```python
from build123d import *

# Parameters (mm, degrees)
SALIENTE_EXTRUIR1_DEPTH = 6


with BuildPart() as part:
    # Corte → Saliente-Extruir1 (new body)
    with BuildSketch(Plane.XY):
        Polygon((113.99992211, 146.05), (113.999928646, 140), (86.000028142, 140), (86.000028142, 146.05), (80.000028142, 146.05), (80.000028142, 140), (76.000028142, 140), (76.000028142, 131.000000972), (75.000028142, 130.000001013), (57.20005465, 130.000001734), (56.20005465, 129.000001774), (56.20005465, 71.000001774), (57.20005465, 70.000001734), (75.000028142, 70.000001013), (76.000028142, 69.000000972), (76.000028142, 60), (80.000028142, 60), (80.000028142, 53.95), (86.000028142, 53.95), (86.000028142, 60), (114.00001507, 60), (114.000021606, 53.95), (120.000021606, 53.95), (120.00001507, 60), (124.00001507, 60), (124.000005347, 68.999999028), (125.000004267, 69.999998987), (142.80005465, 69.999998266), (143.80005465, 70.999998226), (143.80005465, 128.999998226), (142.80005465, 129.999998266), (124.999939449, 129.999998987), (123.999938369, 130.999999028), (123.999928646, 140), (119.999928646, 140), (119.99992211, 146.05), align=None)
        Polygon((71.50005465, 126.700001641), (128.50005465, 126.699998845), (128.50005465, 120.699998845), (71.50005465, 120.700001155), align=None, mode=Mode.SUBTRACT)
        Polygon((87.50005465, 73.300000506), (128.50005465, 73.299998359), (128.50005465, 79.299998845), (87.50005465, 79.300000506), align=None, mode=Mode.SUBTRACT)
        with BuildLine():
            add(Edge.make_bspline(
                [(139.147057668, 90.199998471), (139.147059335, 89.428473471), (138.521585686, 88.802997119), (137.750060686, 88.802995452)],
                knots=[0, 0, 0, 0, 1, 1, 1, 1], degree=3))
            add(Edge.make_bspline(
                [(137.750060686, 88.802995452), (136.978535686, 88.802993785), (136.353059335, 89.428467434), (136.353057668, 90.199992434)],
                knots=[0, 0, 0, 0, 1, 1, 1, 1], degree=3))
            add(Edge.make_bspline(
                [(136.353057668, 90.199992434), (136.353056001, 90.971517434), (136.97852965, 91.596993785), (137.75005465, 91.596995452)],
                knots=[0, 0, 0, 0, 1, 1, 1, 1], degree=3))
            add(Edge.make_bspline(
                [(137.75005465, 91.596995452), (138.52157965, 91.596997119), (139.147056001, 90.971523471), (139.147057668, 90.199998471)],
                knots=[0, 0, 0, 0, 1, 1, 1, 1], degree=3))
        make_face(mode=Mode.SUBTRACT)
        with BuildLine():
            add(Edge.make_bspline(
                [(139.147057668, 121.799998471), (139.147059335, 121.028473471), (138.521585686, 120.402997119), (137.750060686, 120.402995452)],
                knots=[0, 0, 0, 0, 1, 1, 1, 1], degree=3))
            add(Edge.make_bspline(
                [(137.750060686, 120.402995452), (136.978535686, 120.402993785), (136.353059335, 121.028467434), (136.353057668, 121.799992434)],
                knots=[0, 0, 0, 0, 1, 1, 1, 1], degree=3))
            add(Edge.make_bspline(
                [(136.353057668, 121.799992434), (136.353056001, 122.571517434), (136.97852965, 123.196993785), (137.75005465, 123.196995452)],
                knots=[0, 0, 0, 0, 1, 1, 1, 1], degree=3))
            add(Edge.make_bspline(
                [(137.75005465, 123.196995452), (138.52157965, 123.196997119), (139.147056001, 122.571523471), (139.147057668, 121.799998471)],
                knots=[0, 0, 0, 0, 1, 1, 1, 1], degree=3))
        make_face(mode=Mode.SUBTRACT)
        with BuildLine():
            add(Edge.make_bspline(
                [(63.647057668, 121.800001529), (63.647059335, 121.028476529), (63.021585686, 120.403000178), (62.250060686, 120.402998511)],
                knots=[0, 0, 0, 0, 1, 1, 1, 1], degree=3))
            add(Edge.make_bspline(
                [(62.250060686, 120.402998511), (61.478535686, 120.402996844), (60.853059335, 121.028470493), (60.853057668, 121.799995493)],
                knots=[0, 0, 0, 0, 1, 1, 1, 1], degree=3))
            add(Edge.make_bspline(
                [(60.853057668, 121.799995493), (60.853056001, 122.571520493), (61.47852965, 123.196996844), (62.25005465, 123.196998511)],
                knots=[0, 0, 0, 0, 1, 1, 1, 1], degree=3))
            add(Edge.make_bspline(
                [(62.25005465, 123.196998511), (63.02157965, 123.197000178), (63.647056001, 122.571526529), (63.647057668, 121.800001529)],
                knots=[0, 0, 0, 0, 1, 1, 1, 1], degree=3))
        make_face(mode=Mode.SUBTRACT)
        with BuildLine():
            add(Edge.make_bspline(
                [(63.647057668, 90.200001529), (63.647059335, 89.428476529), (63.021585686, 88.803000178), (62.250060686, 88.802998511)],
                knots=[0, 0, 0, 0, 1, 1, 1, 1], degree=3))
            add(Edge.make_bspline(
                [(62.250060686, 88.802998511), (61.478535686, 88.802996844), (60.853059335, 89.428470493), (60.853057668, 90.199995493)],
                knots=[0, 0, 0, 0, 1, 1, 1, 1], degree=3))
            add(Edge.make_bspline(
                [(60.853057668, 90.199995493), (60.853056001, 90.971520493), (61.47852965, 91.596996844), (62.25005465, 91.596998511)],
                knots=[0, 0, 0, 0, 1, 1, 1, 1], degree=3))
            add(Edge.make_bspline(
                [(62.25005465, 91.596998511), (63.02157965, 91.597000178), (63.647056001, 90.971526529), (63.647057668, 90.200001529)],
                knots=[0, 0, 0, 0, 1, 1, 1, 1], degree=3))
        make_face(mode=Mode.SUBTRACT)
    extrude(amount=-SALIENTE_EXTRUIR1_DEPTH)


solid = part.part
```
The model under review builds one solid part; all positions refer to its coordinate system, in mm. A direction names the side the tool comes from. Round coordinates to 2 decimals unless told otherwise and drop trailing zeros. Loops run counter-clockwise (first coordinate to the right, second up) from the corner with the lowest first, then second, coordinate; pieces in that order, holes last. Notation, with made-up numbers: M -38,54.5 L 17,54.5 A21 ccw 17,59.5 Z; hole C 66,33 d8. An arc over 180 degrees is marked long. Answer as a JSON object with one key per item and string values.
(1) To check wall thickness, follow line 1 along Y through (x, z) = (62, -5.5); line 2 along Y through (x, z) = (108.5, -1.5); line 3 along Y through (x, z) = (81, -1.75). State the ranges of each line that lie inside material, in increasing order.
Resolved:
{"line 1": "70 to 88.83, 91.57 to 120.43, 123.17 to 130", "line 2": "60 to 73.3, 79.3 to 120.7, 126.7 to 140", "line 3": "53.95 to 120.7, 126.7 to 146.05"}
(2) Clearance check with flat-ended pins moving along their axes: P1, Ø1.8, axis at x = 107.5, z = -3.5, coming from the +Y side; P2, Ø3, axis at y = 56, z = -2.5, coming from the -X side; P3, Ø2, axis at y = 136.5, z = -1.5, coming from the +X side. State where each tip first meets the part, or that it passes through.
Resolved:
{"P1": "y = 140", "P2": "x = 80", "P3": "x = 124"}
(3) Take a section at D-D on y = 138. Give the boundary of the cut face in (x, z).
Resolved:
{"outline": "M 76,-6 L 124,-6 L 124,0 L 76,0 Z"}
(4) Take a section at B-B on x = 102.5. Give the boundary of the cut face in (y, z), and give its area (3 significant figures).
Resolved:
{"outline": "M 60,-6 L 73.3,-6 L 73.3,0 L 60,0 Z; M 79.3,-6 L 120.7,-6 L 120.7,0 L 79.3,0 Z; M 126.7,-6 L 140,-6 L 140,0 L 126.7,0 Z", "area": "408 mm²"}
(5) Take a section at A-A on y = 78. Give the boundary of the cut face in (x, z), and give its area (3 significant figures).
Resolved:
{"outline": "M 56.2,-6 L 87.5,-6 L 87.5,0 L 56.2,0 Z; M 128.5,-6 L 143.8,-6 L 143.8,0 L 128.5,0 Z", "area": "280 mm²"}
(6) Take a section at C-C on x = 69.5. Give the boundary of the cut face in (y, z), and give its area (3 significant figures).
Resolved:
{"outline": "M 70,-6 L 130,-6 L 130,0 L 70,0 Z", "area": "360 mm²"}
(7) Tool access review of faces 1 (the flat face through (86, 143, -3)), 2 (the flat face through (76, 136, -3)), 3 (the flat face through (78, 60, -3)), 4 (the flat face through (108, 79.3, -3)): name each direction out of +Z, -Z, +X, -X, +Y, -Y from which nothing blocks a thin tool from reaching the whole face with its end or side.
Resolved:
{"face 1": "+Z, -Z, +Y", "face 2": "+Z, -Z, -X, +Y", "face 3": "+Z, -Z, -X, -Y", "face 4": "+Z, -Z"}
